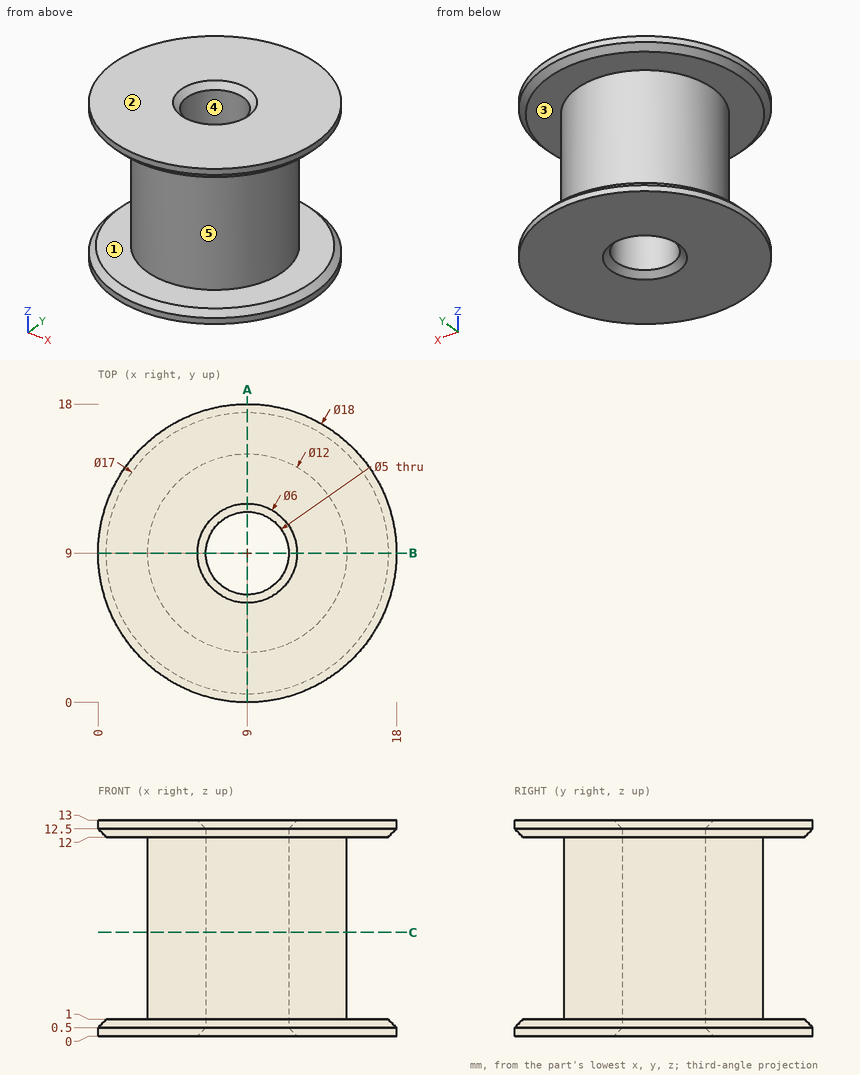
Study the drawing (mm; zero at the part's minimum x, y, z) and answer. A direction names the side the tool comes from. Round coordinates to 2 decimals unless told otherwise and drop trailing zeros. Order: outer loops, then holes, each group sorted by start corner. A loop starts at its lowest first (then second) coordinate and runs counter-clockwise, first axis right, second up. Notation, with made-up numbers: M 81.5,-15 L 95.5,-15 A21 ccw 95.5,11 Z; hole C 58.25,-20 d1. An arc over 180 degrees is marked long. One line per item, written item: value.
Q1. For the marked faces 1 and 2, determine the directions among +Z, -Z, +X, -X, +Y, -Y from which every point of the face is accessible in a straight line to the end or side of a thin tool.
Derived:
face 1: none
face 2: +Z, +X, -X, +Y, -Y
Q2. Flat-ended cylindrical pins translate along their axes: pin 1 (3 mm diameter, centred on y = 11, z = 7, fed in from +X); pin 2 (1 mm diameter, centred on x = 3, z = 4.5, fed in from +Y); pin 3 (4 mm diameter, centred on x = 4.5, z = 4.5, fed in from -Y). Find the tip coordinate at first contact, or state that the pin passes through.
Derived:
pin 1: x = 14.98
pin 2: y = 11.4
pin 3: y = 3.55
Q3. Find section A-A on x = 9. Write down the section's boundary in (y, z).
Derived:
outline: M 0,0 L 6,0 L 6.5,0.5 L 6.5,12.5 L 6,13 L 0,13 L 0,12.5 L 0.5,12 L 3,12 L 3,1 L 0.5,1 L 0,0.5 Z; M 11.5,0.5 L 12,0 L 18,0 L 18,0.5 L 17.5,1 L 15,1 L 15,12 L 17.5,12 L 18,12.5 L 18,13 L 12,13 L 11.5,12.5 Z
Q4. Determine the mould class of the marked faces 3, 4 and 5 for opening direction Y: released by +Y, released by -Y, zero draft, split by the parting line, or undercut.
Derived:
face 3: zero draft
face 4: undercut
face 5: split by the parting line
Q5. Straight lines are drawn through the part: line 1 (Z direction, x = 11.25, y = 2); line 2 (Y direction, x = 9, z = 4.75); line 3 (Y direction, x = 7, z = 9). For each, find the intervals that lie inside material, in ascending order.
Derived:
line 1: 0 to 1, 12 to 13
line 2: 3 to 6.5, 11.5 to 15
line 3: 3.34 to 7.5, 10.5 to 14.66
Q6. Find section C-C on z = 6.25. Write down the section's boundary in (x, y).
Derived:
outline: C 9,9 d12; hole C 9,9 d5
